Part model, mm, in its own coordinate system. A direction names the side the tool comes from. Give positions to 0.01 mm unless a question says otherwise; leave off trailing zeros. Order: outer loops, then holes, each group sorted by start corner. A loop starts at its lowest first (then second) coordinate and runs counter-clockwise, first axis right, second up.
1. Slice it at B-B on y = -43. List the corners of the cut face in (x, z).
2. Probe line 1 (Z direction, x = 60, y = -42.25); line 2 (Y direction, x = 21, z = 6.25); line 3 (X direction, y = 47, z = 10). List the from-to ranges inside material, lowest first.
3. Slice it at A-A on x = 37.5. List the corners of the cut face in (y, z), and give its area (3 significant figures).
4. Mould opens along X. For faces 3 (the cylindrical face through (57.253, 44.57, 9.879)), 4 (the flat face through (-10, -1, 10)), 5 (the flat face through (35, -39.5, 10)), 6 (the cylindrical face through (57.253, -44.43, 9.879)) say: +X half, -X half, draft (parallel to the pull), parting line (faces both ways), or undercut.
5. Drop flat-ended pins along their axis: pin 1 Ø2 at (y, z) = (25.5, 15.5) entering from +X; pin 2 Ø10 at (y, z) = (39, 16.5) entering from +X. Give the stop position or say it passes through.
6. Slice it at C-C on y = -22. List the corners of the cut face in (x, z), and give its area (3 significant figures).
7. Which spindle directions (+Z, -Z, +X, -X, +Y, -Y) get a long thin tool onto all of the face, cutting with end or side? Do faces 1 (the flat face through (0, 1, 10)), 2 (the flat face through (31, -49.5, 10)). Say none if no direction does.
from build123d import *

# Parameters (mm, degrees)
EXTRUDE_1_DEPTH     = 20
CUT_EXTRUDE_1_DEPTH = 123.886126149


with BuildPart() as part:
    # 草图1 → 凸台-拉伸1 (new body)
    with BuildSketch(Plane.XY):
        Polygon((0, 39.5), (0, -39.5), (70, -39.5), (70, -49.5), (-10, -49.5), (-10, 49.5), (70, 49.5), (70, 39.5), align=None)
    extrude(amount=EXTRUDE_1_DEPTH)

    # 草图2 → 切除-拉伸1 (cut, through all)
    with BuildSketch(Plane(origin=(0, 49.5, 0), x_dir=(1, 0, 0), z_dir=(0, 1, 0))):
        with BuildLine():
            ThreePointArc((57.25, -10), (60, -12.75), (62.75, -10))
            Line((62.75, -10), (57.25, -10))
        make_face()
        with BuildLine():
            Line((57.25, -10), (62.75, -10))
            ThreePointArc((62.75, -10), (60, -7.25), (57.25, -10))
        make_face()
        with BuildLine():
            ThreePointArc((60, 0), (67.071067812, -2.928932188), (70, -10))
            Line((70, -10), (70, 0))
            Line((70, 0), (60, 0))
        make_face()
        with BuildLine():
            Line((70, -20), (70, -10))
            ThreePointArc((70, -10), (67.071067812, -17.071067812), (60, -20))
            Line((60, -20), (70, -20))
        make_face()
    extrude(amount=-CUT_EXTRUDE_1_DEPTH, mode=Mode.SUBTRACT)


solid = part.part
Data:
1. outline: (-10, 0) - (60, 0) arc R10 ccw to (60, 20) - (-10, 20) - close; hole circle Ø5.5 at (60, 10)
2. line 1: z = 0 to 7.25, 12.75 to 20
2. line 2: y = -49.5 to -39.5, 39.5 to 49.5
2. line 3: x = -10 to 57.25, 62.75 to 70
3. outline: (-49.5, 0) - (-39.5, 0) - (-39.5, 20) - (-49.5, 20) - close; (39.5, 0) - (49.5, 0) - (49.5, 20) - (39.5, 20) - close
3. area: 400 mm2
4. face 3: undercut
4. face 4: -X half
4. face 5: draft
4. face 6: undercut
5. pin 1: stops at x = 0
5. pin 2: stops at x = 69.88
6. outline: (-10, 0) - (0, 0) - (0, 20) - (-10, 20) - close
6. area: 200 mm2
7. face 1: +Z, -Z, +X
7. face 2: +Z, -Z, +X, -X, -Y
